Geometry: final body of the model. Coordinates: model frame, mm. Give positions to 0.01 mm unless a question says otherwise; leave off trailing zeros. Order: outer loops, then holes, each group sorted by start corner. A loop starts at its lowest first (then second) coordinate and runs counter-clockwise, first axis right, second up. Notation, with made-up numbers: (39.25, 1) - (83.25, 1) arc R32 ccw to (83.25, 36) - close; hole circle Ø3 at (34.5, 88). An arc over 180 degrees is marked (long way). Put each result on its own line as item: value. Start each with the question number.
1. First-contact query: P1, Ø8, axis at y = 10, z = 75.5, coming from the +X side; P2, Ø7, axis at x = 0, z = 0, coming from the -Y side; P3, Ø12, axis at y = 17.5, z = 257, coming from the -X side; P4, Ø1.5, axis at y = 7, z = 86.5, coming from the +X side. Flat tips, straight axial feed; report the tip coordinate or a pass-through.
2. Section A-A on z = 0. Return the cut outline in (x, y), plus the area to 3 significant figures.
3. Section C-C on x = 0. Return the cut outline in (y, z), plus the area to 3 significant figures.
4. Ray query, line 1 along X through (y, z) = (11.25, 0); line 2 along Z through (x, y) = (0, 14.25); line 3 along Z through (x, y) = (0.5, 8.5). Return the intervals inside material, ascending. Write a range as from..to.
5. Section B-B on y = 13.5. Return the cut outline in (x, z), plus the area to 3 significant figures.
6. Section D-D on z = 55.5. Return the cut outline in (x, y).
from build123d import *

# Parameters (mm, degrees)
BOSS_EXTRUDE2_DEPTH = 20
SKETCH3_R           = 5.75
CUT_EXTRUDE1_DEPTH  = 21


with BuildPart() as part:
    # Sketch2 → Boss-Extrude2 (new body)
    with BuildSketch(Plane(origin=(0, 0, 0), x_dir=(1, 0, 0), z_dir=(0, 1, 0))):
        Polygon((-12.666179626, 10), (-12.666179626, -15), (198.957090302, -312.389629316), (198.957090302, -332.698194406), (224.289449554, -332.698194406), (224.289449554, -312.389629316), (12.666179626, -15), (12.666179626, 10), align=None)
    extrude(amount=BOSS_EXTRUDE2_DEPTH)

    # Sketch3 → Cut-Extrude1 (cut, through all)
    with BuildSketch(Plane(origin=(0, 20, 0), x_dir=(1, 0, 0), z_dir=(0, 1, 0))):
        Circle(SKETCH3_R)
        with Locations((210.164682847, -318.99029152)):
            Circle(SKETCH3_R)
    extrude(amount=-CUT_EXTRUDE1_DEPTH, mode=Mode.SUBTRACT)


solid = part.part
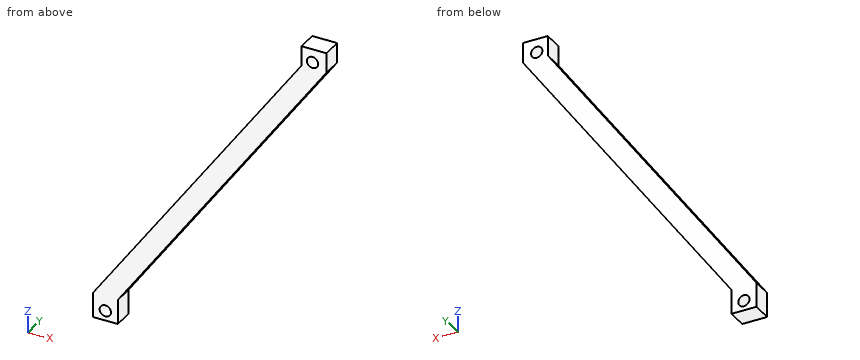
Resolved:
1. P1: x = 58.56
1. P2: through
1. P3: x = 155.27
1. P4: x = 64.08
2. outline: (-12.67, 0) - (-5.75, 0) - (-5.75, 20) - (-12.67, 20) - close; (5.75, 0) - (12.67, 0) - (12.67, 20) - (5.75, 20) - close
2. area: 277 mm^2
3. outline: (0, -10) - (20, -10) - (20, -5.75) - (0, -5.75) - close; (0, 5.75) - (20, 5.75) - (20, 32.8) - (0, 32.8) - close
3. area: 626 mm^2
4. line 1: -12.67..-5.75, 5.75..12.67
4. line 2: -10..-5.75, 5.75..32.8
4. line 3: -10..-5.73, 5.73..33.5
5. outline: (-12.67, -10) - (12.67, -10) - (12.67, 15) - (224.29, 312.39) - (224.29, 332.7) - (198.96, 332.7) - (198.96, 312.39) - (-12.67, 15) - close; hole circle Ø11.5 at (0, 0); hole circle Ø11.5 at (210.16, 318.99)
5. area: 8,470 mm^2
6. outline: (16.15, 0) - (41.49, 0) - (41.49, 20) - (16.15, 20) - close
